Answer from the drawing. Dimensions are ordinates in mm from the lowest x, y and z of the part. A direction names the side the tool comes from. Round coordinates to 2 decimals unless told otherwise and drop trailing zeros. Write each loop counter-clockwise with the first axis right and the second up, starting at its lowest first coordinate (ties: lowest second). Pieces come first, ordered by that corner, then holes. Notation, with made-up numbers: (85, 2) -> (139, 2) arc R26 ccw to (139, 38) -> close; hole circle Ø7 at (-29, -3). An arc over 180 degrees is marked (long way). Answer as a JSON object with one key per item and string values. Group by question number.
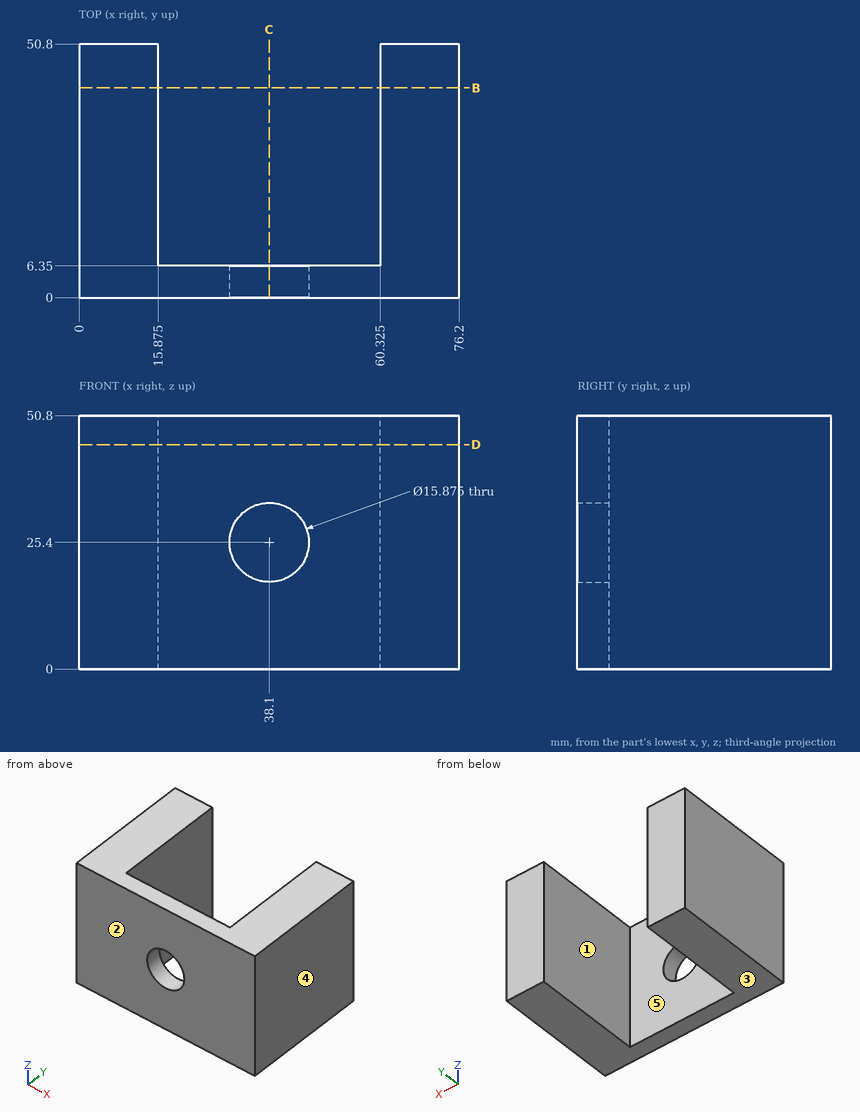
1) Each of these flat-tipped pins is pushed along its axis until it touches: P1, Ø8, axis at x = 49, z = 29, coming from the +Y side; P2, Ø2, axis at x = 42, z = 29, coming from the -Y side. Where does it stop, or does it pass through?
2) A cutting plane is placed at D-D on z = 45. Determine the outline of the cut face in (x, y) (3 decimals), plus the area to 3 significant figures.
3) A tool of negligible diameter and unlimited length cuts with its end or side. For the marked faces 1 and 2, from which of +Z, -Z, +X, -X, +Y, -Y can it reach the whole face along a straight path? Write none if from no direction.
4) For a pull along X with two mould halves and no side action, classify the marked faces 3, 4 and 5 as released by +X, released by -X, zero draft, split by the parting line, or undercut.
5) A cutting plane is placed at C-C on x = 38.1. Determine the outline of the cut face in (y, z), plus the area to 3 significant figures.
6) Straight lines are drawn through the part: L1, parallel to X at y = 47, z = 38.5 (3 decimals); L2, parallel to Z at x = 38, y = 1; L3, parallel to X at y = 2.5, z = 25.4. For each, find the intervals that lie inside material, in ascending order.
7) A cutting plane is placed at B-B on y = 42. Determine the outline of the cut face in (x, z) (3 decimals), plus the area to 3 significant figures.
Established:
{
 "1": {"P1": "stops at y = 6.35", "P2": "passes through"},
 "2": {"outline": "(0, 0) -> (76.2, 0) -> (76.2, 50.8) -> (60.325, 50.8) -> (60.325, 6.35) -> (15.875, 6.35) -> (15.875, 50.8) -> (0, 50.8) -> close", "area": "1,900 mm²"},
 "3": {"face 1": "+Z, -Z, +Y", "face 2": "+Z, -Z, +X, -X, -Y"},
 "4": {"face 3": "zero draft", "face 4": "released by +X", "face 5": "undercut"},
 "5": {"outline": "(0, 0) -> (6.35, 0) -> (6.35, 17.46) -> (0, 17.46) -> close; (0, 33.34) -> (6.35, 33.34) -> (6.35, 50.8) -> (0, 50.8) -> close", "area": "222 mm²"},
 "6": {"L1": "x = 0 to 15.875, 60.325 to 76.2", "L2": "z = 0 to 17.46, 33.34 to 50.8", "L3": "x = 0 to 30.16, 46.04 to 76.2"},
 "7": {"outline": "(0, 0) -> (15.875, 0) -> (15.875, 50.8) -> (0, 50.8) -> close; (60.325, 0) -> (76.2, 0) -> (76.2, 50.8) -> (60.325, 50.8) -> close", "area": "1,610 mm²"}
}
